For this review, take the finished solid that the model builds, in its own axes (mm). A direction names the side the tool comes from. Give positions to 0.01 mm unless a question says otherwise; leave off trailing zeros. Loops run counter-clockwise (first coordinate to the right, second up) from the corner with the lowest first, then second, coordinate; pieces in that order, holes last. Notation, with made-up numbers: (5, -31) -> (25, -31) arc R20 ccw to (25, -25) -> close; hole circle Ø1 at (-11.5, 53.25). An arc over 180 degrees is marked (long way). Write each question's results on one line, items separated by ' | '. Start each with the question number.
```python
from build123d import *

# Parameters (mm, degrees)
F2_SIZE  = 0.5
F3_SIZE  = 0.7
F5_DEPTH = 2.5


with BuildPart() as f1:
    # F0 (on Front) → F1 (revolve)
    with BuildSketch(Plane.XZ):
        Polygon((3, 2.5), (1.5, 2.5), (1.5, 7), (0, 7), (0, -20), (2, -20), (2, 0), (3, 0), align=None)
    revolve(axis=Axis((0, 0, -6.5), (0, 0, 1)))

    # F2
    f2_edges = [f1.edges().sort_by_distance(p)[0] for p in [
        (-1.5, 0, 7),
    ]]
    chamfer(f2_edges, length=F2_SIZE)

    # F3
    f3_edges = [f1.edges().sort_by_distance(p)[0] for p in [
        (-2, 0, -20),
    ]]
    chamfer(f3_edges, length=F3_SIZE)

    # F4 (on face) → F5 (cut, through all)
    with BuildSketch(Plane(origin=(0, 0, 0), x_dir=(1, 0, 0), z_dir=(0, 0, -1))):
        with BuildLine():
            ThreePointArc((3, 0), (2.8722813233, 0.8660254038), (2.5, 1.6583123952))
            Line((2.5, 1.6583123952), (2.5, -1.6583123952))
            ThreePointArc((2.5, -1.6583123952), (2.8722813233, -0.8660254038), (3, 0))
        make_face()
        with BuildLine():
            Line((-2.5, -1.6583123952), (-2.5, 1.6583123952))
            ThreePointArc((-2.5, 1.6583123952), (-3, 0), (-2.5, -1.6583123952))
        make_face()
    extrude(amount=-F5_DEPTH, mode=Mode.SUBTRACT)


solid = f1.part
```
1. We need section C-C (z = 0.25). Write out the cut boundary in (x, y), plus the area to 3 significant figures.
2. We need section D-D (z = -10.25). Write out the cut boundary in (x, y).
3. For pin 1 Ø2 at (y, z) = (2, -4) entering from +X; pin 2 Ø2 at (x, y) = (1.5, 2) entering from -Z; pin 3 Ø2 at (x, y) = (-2, -0.5) entering from -Z, all flat-tipped, find the tip position at first contact; note any pin that passes through.
4. We need section A-A (x = 0). Write out the cut boundary in (y, z), plus the area to 3 significant figures.
5. We need section B-B (y = 0). Write out the cut boundary in (x, z).
6. Machinability: for faces 1 (the flat face through (2, 0, 2.5)), 2 (the cylindrical face through (0, -2, -10)), 3 (the flat face through (0, 0, 7)), which of the approach directions +Z, -Z, +X, -X, +Y, -Y give a long, thin tool a straight path to every point of the face, cutting with its end or side? Answer none if there is none.
7. Wall thickness on L1, parallel to Y at x = 0, z = -11.75; L2, parallel to Z at x = 1.65, y = 1.8; L3, parallel to X at y = -0.35, z = -11.75: over which ranges is each line inside the solid? List them lowest first.
Response:
1) outline: (-2.5, -1.66) arc R3 ccw to (2.5, -1.66) -> (2.5, 1.66) arc R3 ccw to (-2.5, 1.66) -> close | area: 26.0 mm2
2) outline: circle Ø4 at (0, 0)
3) pin 1: stops at x = 1.73 | pin 2: stops at z = -19.8 | pin 3: stops at z = -20
4) outline: (-3, 0) -> (-2, 0) -> (-2, -19.3) -> (-1.3, -20) -> (1.3, -20) -> (2, -19.3) -> (2, 0) -> (3, 0) -> (3, 2.5) -> (1.5, 2.5) -> (1.5, 6.5) -> (1, 7) -> (-1, 7) -> (-1.5, 6.5) -> (-1.5, 2.5) -> (-3, 2.5) -> close | area: 108 mm2
5) outline: (-2.5, 0) -> (-2, 0) -> (-2, -19.3) -> (-1.3, -20) -> (1.3, -20) -> (2, -19.3) -> (2, 0) -> (2.5, 0) -> (2.5, 2.5) -> (1.5, 2.5) -> (1.5, 6.5) -> (1, 7) -> (-1, 7) -> (-1.5, 6.5) -> (-1.5, 2.5) -> (-2.5, 2.5) -> close
6) face 1: +Z | face 2: -Z | face 3: +Z, +X, -X, +Y, -Y
7) L1: y = -2 to 2 | L2: z = 0 to 2.5 | L3: x = -1.97 to 1.97
